```python
from build123d import *

# Parameters (mm, degrees)
F1_DEPTH = 7


with BuildPart() as f1:
    # F0 (on Right) → F1 (new body)
    with BuildSketch(Plane.YZ):
        with BuildLine():
            Line((-57.826925, -19.807692), (-57.826925, 20.192308))
            Line((-57.826925, 20.192308), (-49.826925, 20.192308))
            Line((-49.826925, 20.192308), (-49.826925, -19.807692))
            Line((-49.826925, -19.807692), (-40.826925, -19.807692))
            Line((-40.826925, -19.807692), (-40.826925, 40.192308))
            Line((-40.826925, 40.192308), (-39.828869, 159.95899))
            Line((-39.828869, 159.95899), (-39.826925, 160.192308))
            ThreePointArc((-39.826925, 160.192308), (-53.826925, 174.192308), (-67.826925, 160.192308))
            Line((-67.826925, 160.192308), (-67.82498, 159.95899))
            Line((-67.82498, 159.95899), (-66.826925, 40.192308))
            Line((-66.826925, 40.192308), (-66.826925, -19.807692))
            Line((-66.826925, -19.807692), (-57.826925, -19.807692))
        make_face()
        with BuildLine():
            ThreePointArc((-42.826925, 160.192308), (-46.04875, 152.414133), (-53.826925, 149.192308))
            ThreePointArc((-53.826925, 149.192308), (-61.605099, 152.414133), (-64.826925, 160.192308))
            ThreePointArc((-64.826925, 160.192308), (-53.826925, 171.192308), (-42.826925, 160.192308))
        make_face(mode=Mode.SUBTRACT)
    extrude(amount=F1_DEPTH)


solid = f1.part
```
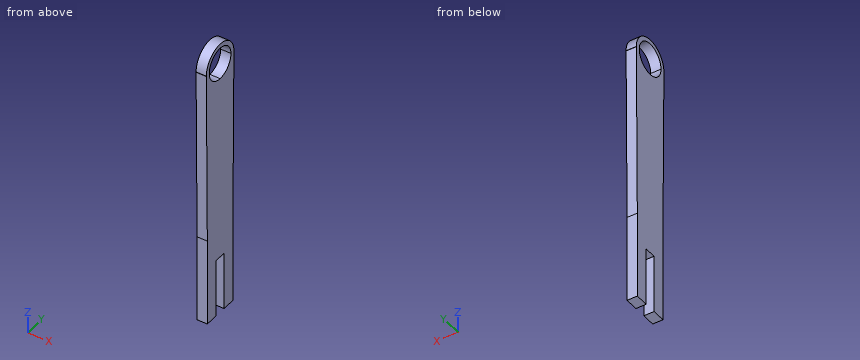
Can you work these out from the model? Positions are in its coordinate system, mm. Coordinates: 2 decimals unless noted, no trailing zeros. Loops run counter-clockwise (first coordinate to the right, second up) from the corner with the lowest first, then second, coordinate; pieces in that order, holes last. Notation, with made-up numbers: (-14.5, 2.25) - (43.5, 2.25) arc R17 cw to (43.5, 28.25) - close; hole circle Ø9 at (43.25, -27). An arc over 180 degrees is marked (long way). Answer as CSV lines item,"result". Start each with the question number.
1) For pin 1 (4 mm diameter, centred on y = -60, z = 109, fed in from -X); pin 2 (2 mm diameter, centred on x = 3.5, y = -54, fed in from -Z); pin 3 (2 mm diameter, centred on x = 3, z = -9.5, fed in from -Y); pin 4 (3 mm diameter, centred on x = 2.5, z = 94.5, fed in from +Y), each with a flat end and sliding along its axis, tell me the tip position at first contact or that it passes through.
2) I need wall thicknesses on line 1 (Z direction, x = 2.5, y = -53.5); line 2 (Y direction, x = 2.5, z = 5); line 3 (Y direction, x = 0.5, z = 154). Which ranges of each line are inside material? Lowest first, please. Write a range as from..to.
3) Suppose I cut it at A-A (y = -46.25). Please give me the cut outline in (x, z).
4) Suppose I cut it at C-C (z = 155). Please give me the cut outline in (x, y), plus the area to 3 significant figures.
5) Suppose I cut it at B-B (x = 4). Please give me the cut outline in (y, z), plus the area to 3 significant figures.
6) Suppose I cut it at D-D (z = 54.5). Please give me the cut outline in (x, y), plus the area to 3 significant figures.
Check result:
1,pin 1,"stops at x = 0"
1,pin 2,"stops at z = 20.19"
1,pin 3,"stops at y = -66.83"
1,pin 4,"stops at y = -40.36"
2,line 1,"z = 20.19..149.2, 171.19..174.19"
2,line 2,"y = -66.83..-57.83, -49.83..-40.83"
2,line 3,"y = -67.78..-62.92, -44.74..-39.88"
3,outline,"(0, -19.81) - (7, -19.81) - (7, 152.22) - (0, 152.22) - close; (0, 168.17) - (7, 168.17) - (7, 171.96) - (0, 171.96) - close"
4,outline,"(0, -67.78) - (7, -67.78) - (7, -63.52) - (0, -63.52) - close; (0, -44.13) - (7, -44.13) - (7, -39.87) - (0, -39.87) - close"
4,area,"59.6 mm²"
5,outline,"(-67.83, 160.19) - (-67.82, 159.96) - (-66.83, 40.19) - (-66.83, -19.81) - (-57.83, -19.81) - (-57.83, 20.19) - (-49.83, 20.19) - (-49.83, -19.81) - (-40.83, -19.81) - (-40.83, 40.19) - (-39.83, 159.96) - (-39.83, 160.19) arc R14 ccw to start; hole (-53.83, 149.19) arc R11 ccw to (-42.83, 160.19) arc R11 ccw (long way) to start"
5,area,"4,410 mm²"
6,outline,"(0, -66.95) - (7, -66.95) - (7, -40.71) - (0, -40.71) - close"
6,area,"184 mm²"
